```python
from build123d import *

# Parameters (mm, degrees)
F2_DEPTH = 25.4
F3_DEPTH = 5
F6_D     = 8
F6_DEPTH = 5
F6_TIP   = 2.4034424761
F7_D     = 8
F7_DEPTH = 4
F7_TIP   = 2.4034424761
F8_R     = 3


with BuildPart() as f2:
    # F0 (on Front) → F2 (new body)
    with BuildSketch(Plane.XZ):
        with BuildLine():
            Line((26.353785117, 9.4592816856), (37.6482644529, 13.5132595508))
            ThreePointArc((37.6482644529, 13.5132595508), (30.8672872021, 25.4403337396), (20.4548362885, 34.3744043208))
            Line((20.4548362885, 34.3744043208), (14.3183854019, 24.0620830246))
            ThreePointArc((14.3183854019, 24.0620830246), (21.6071010415, 17.8082336177), (26.353785117, 9.4592816856))
        make_face()
    extrude(amount=F2_DEPTH)

    # F1 (on Front) + F0 (on Front) → F3 (join)
    with BuildSketch(Plane.XZ):
        with BuildLine():
            ThreePointArc((12.2729017731, 20.6246425925), (18.5203723213, 15.2642002437), (22.5889586717, 8.1079557305))
            Line((22.5889586717, 8.1079557305), (37.6482644529, 13.5132595508))
            ThreePointArc((37.6482644529, 13.5132595508), (30.8672872021, 25.4403337396), (20.4548362885, 34.3744043208))
            Line((20.4548362885, 34.3744043208), (12.2729017731, 20.6246425925))
        make_face()
    with BuildSketch(Plane.XZ):
        with BuildLine():
            Line((26.353785117, 9.4592816856), (37.6482644529, 13.5132595508))
            ThreePointArc((37.6482644529, 13.5132595508), (30.8672872021, 25.4403337396), (20.4548362885, 34.3744043208))
            Line((20.4548362885, 34.3744043208), (14.3183854019, 24.0620830246))
            ThreePointArc((14.3183854019, 24.0620830246), (21.6071010415, 17.8082336177), (26.353785117, 9.4592816856))
        make_face()
    extrude(amount=-F3_DEPTH)

    # F6 (one way)
    with BuildSketch(Plane(origin=(29.0515503707, 0, 23.9438319358), x_dir=(0, 1, 0), z_dir=(-0.7716821801, 0, -0.6360083435))):
        with Locations((-4, 0)):
            Circle(F6_D / 2)
    extrude(amount=-F6_DEPTH, mode=Mode.SUBTRACT)
    with Locations(Plane(origin=(29.0515503707, 0, 23.9438319358), x_dir=(0, 1, 0), z_dir=(-0.7716821801, 0, -0.6360083435))):
        with Locations((-4, 0)):
            with Locations((0, 0, -(F6_DEPTH + F6_TIP / 2))):  # 118° drill point
                Cone(0, F6_D / 2, F6_TIP, mode=Mode.SUBTRACT)

    # F7
    with Locations(Plane(origin=(29.0515503707, 0, 23.9438319358), x_dir=(0, 1, 0), z_dir=(0.7716821801, 0, 0.6360083435))):
        with Locations((-4, 0)):
            Hole(F7_D / 2, depth=F7_DEPTH)
            with Locations((0, 0, -(F7_DEPTH + F7_TIP / 2))):  # 118° drill point
                Cone(0, F7_D / 2, F7_TIP, mode=Mode.SUBTRACT)

    # F8
    f8_edges = [f2.edges().sort_by_distance(p)[0] for p in [
        (18.520372, 5, 15.2642),
    ]]
    fillet(f8_edges, radius=F8_R)


solid = f2.part
```
Input: part model. Units: mm. Frame: model coordinates. Coordinates: 2 decimals unless noted, no trailing zeros. Write each loop counter-clockwise with the first axis right and the second up, starting at its lowest first coordinate (ties: lowest second). Pieces come first, ordered by that corner, then holes. Notation, with made-up numbers: (68.5, 86) -> (104.5, 86) arc R28 ccw to (104.5, 108) -> close; hole circle Ø2 at (-34, 28.5). An arc over 180 degrees is marked (long way). Answer as a JSON object with one key per item and string values.
1. Material intervals for line 1 (Y direction, x = 24.5, z = 13); line 2 (Y direction, x = 26.75, z = 20.75); line 3 (X direction, y = -9, z = 23.75), sorted ascending. Write a range as from..to.
Result set:
{"line 1": "y = 0..5", "line 2": "y = -25.4..-7.87, -0.13..5", "line 3": "x = 14.83..32.19"}
2. Section B-B on y = -14.5. Return the cut outline in (x, z).
Result set:
{"outline": "(14.32, 24.06) arc R28 cw to (26.35, 9.46) -> (37.65, 13.51) arc R40 ccw to (20.45, 34.37) -> close"}
3. First-contact query: P1, Ø1, axis at y = -2.5, z = 22.5, coming from the -X side; P2, Ø7, axis at x = 20.5, z = 12.5, coming from the -Y side; P3, Ø6, axis at y = -1, z = 11, coming from the -X side. Flat tips, straight axial feed; report the tip coordinate or a pass-through.
Result set:
{"P1": "stops at x = 15.97", "P2": "stops at y = 0", "P3": "stops at x = 19.62"}
4. Mould query, pull axis X, two halves, no side actions, for faces 1 (the face through (19, 0, 16)), 2 (the face through (24.864, -4.151, 19.613)), 3 (the face through (21.521, -12.522, 17.912)). Classes: released by +X, released by -X, zero draft, split by the parting line, or undercut.
Result set:
{"face 1": "zero draft", "face 2": "undercut", "face 3": "released by -X"}
5. Section A-A on z = 29.5. Return the cut outline in (x, y).
Result set:
{"outline": "(17.55, -25.4) -> (27.01, -25.4) -> (27.01, 5) -> (17.55, 5) -> close"}
